Can you work these out from the model? Positions are in its coordinate system, mm. A direction names the side the tool comes from. Coordinates: 2 decimals unless noted, no trailing zeros. Loops run counter-clockwise (first coordinate to the right, second up) from the corner with the lowest first, then second, coordinate; pieces in that order, holes last. Notation, with made-up numbers: M -26.75,10.5 L 23.25,10.5 A21 ccw 23.25,32.5 Z; hole C -3.5,-15 d3. An arc over 180 degrees is marked long. Answer as a JSON object with one key per item and string values. Group by question number.
Item 1: Suppose I cut it at A-A (y = 19.05). Write out the boundary of the cut face in (x, z) (3 decimals), then the cut area to 3 significant figures.
Item 2: I'm going to push a flat-ended pin straight in: pin 1 Ø4.5 at (x, y) = (31.75, 5.08) entering from +Z. Where does the tip first touch, or does it pass through?
Item 3: Which directions (+Z, -Z, +X, -X, +Y, -Y) give clear straight access to the entire face, cutting with the end or side of a thin tool? Please do faces 4 (the cylindrical face through (70.04, 5.41, 4.1)), 5 (the flat face through (50, 25.4, 3)), 6 (the cylindrical face through (75.54, 23.58, 4.77)), 7 (the cylindrical face through (3.4, 19, 4.9)).
Item 4: If I drill on line 1 (Y direction, x = 31.75, z = 3.75); line 2 (X direction, y = 4.5, z = 0.5); line 3 (X direction, y = 7.75, z = 3.25), over which ranges is the centre line in solid material (lowest first)?
Item 5: Suppose I cut it at D-D (x = 76.2). Write out the boundary of the cut face in (y, z) (3 decimals).
Item 6: Suppose I cut it at B-B (x = 31.75). Write out the boundary of the cut face in (y, z), then the cut area to 3 significant figures.
Item 7: Suppose I cut it at C-C (y = 5.08). Write out the boundary of the cut face in (x, z) (3 decimals).
Item 8: We'd pull the mould along Z, two halves only. Please class faces 1 (the cylindrical face through (85.73, 9.8, 3.13)), 2 (the cylindrical face through (79.748, 5.409, 3.972)), 3 (the flat face through (50, 13, 0)): +Z half, -Z half, draft (parallel to the pull), parting line (faces both ways), or undercut.
```python
from build123d import *

# Parameters (mm, degrees)
SKETCH1_W                           = 101.6
SKETCH1_H                           = 25.4
SKETCH1_R                           = 6.35
SKETCH1_R_2                         = 3.175
BOSS_EXTRUDE1_DEPTH                 = 6.35
F_8_32_TAPPED_HOLE1_REACH           = 105.419
F_8_32_TAPPED_HOLE1_BORE_R          = 1.7272
F_8_32_TAPPED_HOLE1_ON_FACE_2_REACH = 82.385
F_8_32_TAPPED_HOLE1_BORE_2_R        = 1.7272
F_8_32_TAPPED_HOLE2_D               = 3.4544
F_8_32_TAPPED_HOLE2_DEPTH           = 10.668
F_8_32_TAPPED_HOLE2_TIP             = 1.037806461
F_1_4_20_TAPPED_HOLE1_D             = 5.1054


with BuildPart() as part:
    # Sketch1 → Boss-Extrude1 (new body)
    with BuildSketch(Plane.XY):
        with Locations((50.8, 12.7)):
            Rectangle(SKETCH1_W, SKETCH1_H)
        with Locations((92.075, 9.525)):
            Circle(SKETCH1_R, mode=Mode.SUBTRACT)
        with Locations((9.525, 19.05)):
            Circle(SKETCH1_R_2, mode=Mode.SUBTRACT)
        with Locations((76.2, 19.05)):
            Circle(SKETCH1_R_2, mode=Mode.SUBTRACT)
    extrude(amount=BOSS_EXTRUDE1_DEPTH)

    # #8-32 Tapped Hole1 bore (on position points) → #8-32 Tapped Hole1 (cut, up to next)
    with BuildSketch(Plane(origin=(0, 19.05, 3.175), x_dir=(0, 0, -1), z_dir=(-1, 0, 0)), mode=Mode.PRIVATE) as f_8_32_tapped_hole1_sk1:
        Circle(F_8_32_TAPPED_HOLE1_BORE_R)
    f_8_32_tapped_hole1_tool1 = extrude(f_8_32_tapped_hole1_sk1.sketch, amount=-F_8_32_TAPPED_HOLE1_REACH, mode=Mode.PRIVATE) & part.part
    add(f_8_32_tapped_hole1_tool1.solids().sort_by_distance((0, 19.05, 3.175))[0], mode=Mode.SUBTRACT)

    # #8-32 Tapped Hole1 bore 2 (on position points) → #8-32 Tapped Hole1 on face 2 (cut, up to next)
    with BuildSketch(Plane(origin=(76.2, 25.4, 3.175), x_dir=(0, 0, 1), z_dir=(0, 1, 0)), mode=Mode.PRIVATE) as f_8_32_tapped_hole1_on_face_2_sk1:
        Circle(F_8_32_TAPPED_HOLE1_BORE_2_R)
    f_8_32_tapped_hole1_on_face_2_tool1 = extrude(f_8_32_tapped_hole1_on_face_2_sk1.sketch, amount=-F_8_32_TAPPED_HOLE1_ON_FACE_2_REACH, mode=Mode.PRIVATE) & part.part
    add(f_8_32_tapped_hole1_on_face_2_tool1.solids().sort_by_distance((76.2, 25.4, 3.175))[0], mode=Mode.SUBTRACT)

    # #8-32 Tapped Hole2
    with Locations(Plane(origin=(81.28, 0, 3.175), x_dir=(0, 0, -1), z_dir=(0, -1, 0))):
        with Locations((0, 0), (0, -25.4), (0, -68.58), (0, -12.7)):
            Hole(F_8_32_TAPPED_HOLE2_D / 2, depth=F_8_32_TAPPED_HOLE2_DEPTH)
            with Locations((0, 0, -(F_8_32_TAPPED_HOLE2_DEPTH + F_8_32_TAPPED_HOLE2_TIP / 2))):  # 118° drill point
                Cone(0, F_8_32_TAPPED_HOLE2_D / 2, F_8_32_TAPPED_HOLE2_TIP, mode=Mode.SUBTRACT)

    # 1/4-20 Tapped Hole1 (through all)
    with Locations(Plane(origin=(31.75, 5.08, 0), x_dir=(-1, 0, 0), z_dir=(0, 0, -1))):
        with Locations((0, 0)):
            Hole(F_1_4_20_TAPPED_HOLE1_D / 2)


solid = part.part
```
From the geometry:
{
 "1": {"outline": "M 0,0 L 6.35,0 L 6.35,1.448 L 0,1.448 Z; M 0,4.902 L 6.35,4.902 L 6.35,6.35 L 0,6.35 Z; M 12.7,0 L 73.025,0 L 73.025,6.35 L 12.7,6.35 Z; M 79.375,0 L 101.6,0 L 101.6,6.35 L 79.375,6.35 Z", "area": "543 mm2"},
 "2": {"pin 1": "through"},
 "3": {"face 4": "-Y", "face 5": "+Z, -Z, +X, -X, +Y", "face 6": "+Y", "face 7": "-X"},
 "4": {"line 1": "0 to 2.53, 7.63 to 25.4", "line 2": "0 to 29.26, 34.24 to 88.19, 95.96 to 101.6", "line 3": "0 to 10.97, 14.43 to 54.15, 57.61 to 66.85, 70.31 to 79.55, 83.01 to 85.98, 98.17 to 101.6"},
 "5": {"outline": "M 0,0 L 15.875,0 L 15.875,6.35 L 0,6.35 Z; M 22.225,0 L 25.4,0 L 25.4,1.448 L 22.225,1.448 Z; M 22.225,4.902 L 25.4,4.902 L 25.4,6.35 L 22.225,6.35 Z"},
 "6": {"outline": "M 0,0 L 2.53,0 L 2.53,6.35 L 0,6.35 Z; M 7.63,0 L 25.4,0 L 25.4,6.35 L 7.63,6.35 Z", "area": "129 mm2"},
 "7": {"outline": "M 0,0 L 29.197,0 L 29.197,6.35 L 0,6.35 Z; M 34.303,0 L 87.54,0 L 87.54,6.35 L 34.303,6.35 Z; M 96.61,0 L 101.6,0 L 101.6,6.35 L 96.61,6.35 Z; hole C 12.7,3.175 d3.454; hole C 55.88,3.175 d3.454; hole C 68.58,3.175 d3.454; hole C 81.28,3.175 d3.454"},
 "8": {"face 1": "draft", "face 2": "undercut", "face 3": "-Z half"}
}
